from build123d import *

# Parameters (mm, degrees)
SKETCH5_R           = 10
SKETCH5_R_2         = 8.3
BOSS_EXTRUDE1_DEPTH = 15
SKETCH6_R           = 10
BOSS_EXTRUDE2_DEPTH = 2
SKETCH7_W           = 3
SKETCH7_H           = 7
SKETCH7_R           = 0.5
BOSS_EXTRUDE3_DEPTH = 10


with BuildPart() as part:
    # Sketch5 → Boss-Extrude1 (new body)
    with BuildSketch(Plane.XY):
        Circle(SKETCH5_R)
        Circle(SKETCH5_R_2, mode=Mode.SUBTRACT)
    extrude(amount=BOSS_EXTRUDE1_DEPTH)

    # Sketch6 → Boss-Extrude2 (add)
    with BuildSketch(Plane.XY):
        Circle(SKETCH6_R)
    extrude(amount=BOSS_EXTRUDE2_DEPTH)

    # Sketch7 → Boss-Extrude3 (add)
    with BuildSketch(Plane.XY.offset(15)):
        with Locations((0, 13.386859967)):
            Rectangle(SKETCH7_W, SKETCH7_H)
        with Locations((0, 15)):
            Circle(SKETCH7_R, mode=Mode.SUBTRACT)
    extrude(amount=-BOSS_EXTRUDE3_DEPTH)


solid = part.part
Source: CAD feature listing. Evaluate the final solid. Frame: model axes, mm. A direction names the side the tool comes from. Round coordinates to 2 decimals unless told otherwise and drop trailing zeros. Loops run counter-clockwise (first coordinate to the right, second up) from the corner with the lowest first, then second, coordinate; pieces in that order, holes last.
Q1. First-contact query: P1, Ø4, axis at y = -3, z = 9, coming from the -X side; P2, Ø2, axis at x = 5, z = 11.5, coming from the -Y side; P3, Ø8, axis at y = 12, z = 13.5, coming from the -X side. Flat tips, straight axial feed; report the tip coordinate or a pass-through.
Q2. Access query for faces 4 (the face through (1.5, 13, 10)), 5 (the face through (-1.799, -8.103, 8.409)), 6 (the face through (-0.065, 15.496, 10.07)). Directions: +Z, -Z, +X, -X, +Y, -Y. A direction counts if a zero-diameter tool reaches every point of the face in a straight line with its end or side. Return the directions, or none.
Q3. Section C-C, the plane z = 11. Return loops of the section in (x, y).
Q4. Section A-A, the plane y = 15. Return loops of the section in (x, z), plus the area to 3 significant figures.
Q5. Section D-D, the plane y = 0. Return loops of the section in (x, z), plus the area to 3 significant figures.
Q6. Mould query, pull axis Y, two halves, no side actions, for faces 1 (the face through (-2.17, -9.76, 7.4)), 2 (the face through (0, 0, 2)), 3 (the face through (-1.5, 13, 10)). Classes: pulls with the +Y half, pulls with the -Y half, needs draft (parallel to the pull), parting line crosses it, or undercut.
Q7. Section B-B, the plane x = 0. Return loops of the section in (y, z), plus the area to 3 significant figures.
Q8. Ray query, line 1 (Y direction, x = 0, z = 9.75); line 2 (X direction, y = 0, z = 7.5); line 3 (X direction, y = -4.25, z = 13.5). Return the intervals inside material, ascending.
Solutions:
1. P1: stops at x = -9.95
1. P2: stops at y = -9.17
1. P3: stops at x = -6
2. face 4: +Z, -Z, +X, +Y
2. face 5: +Z
2. face 6: +Z, -Z
3. outline: (-1.5, 9.89) arc R10 ccw (long way) to (1.5, 9.89) - (1.5, 16.89) - (-1.5, 16.89) - close; hole circle Ø16.6 at (0, 0); hole circle Ø1 at (0, 15)
4. outline: (-1.5, 5) - (-0.5, 5) - (-0.5, 15) - (-1.5, 15) - close; (0.5, 5) - (1.5, 5) - (1.5, 15) - (0.5, 15) - close
4. area: 20.0 mm2
5. outline: (-10, 0) - (10, 0) - (10, 15) - (8.3, 15) - (8.3, 2) - (-8.3, 2) - (-8.3, 15) - (-10, 15) - close
5. area: 84.2 mm2
6. face 1: parting line crosses it
6. face 2: undercut
6. face 3: needs draft
7. outline: (-10, 0) - (10, 0) - (10, 5) - (14.5, 5) - (14.5, 15) - (8.3, 15) - (8.3, 2) - (-8.3, 2) - (-8.3, 15) - (-10, 15) - close; (15.5, 5) - (16.89, 5) - (16.89, 15) - (15.5, 15) - close
7. area: 143 mm2
8. line 1: y = -10 to -8.3, 8.3 to 14.5, 15.5 to 16.89
8. line 2: x = -10 to -8.3, 8.3 to 10
8. line 3: x = -9.05 to -7.13, 7.13 to 9.05
